```python
from build123d import *

# Parameters (mm, degrees)
F1_DEPTH = 5
F2_R     = 3
F3_DEPTH = 25
F4_SIZE  = 0.6


with BuildPart() as f1:
    # F0 (on Front) → F1 (new body)
    with BuildSketch(Plane.XZ):
        Polygon((2.886751, -5), (5.773503, 0), (2.886751, 5), (-2.886751, 5), (-5.773503, 0), (-2.886751, -5), align=None)
    extrude(amount=F1_DEPTH)

    # F2 (on face) → F3 (join)
    with BuildSketch(Plane.XZ.offset(5)):
        Circle(F2_R)
    extrude(amount=F3_DEPTH)

    # F4
    f4_edges = [f1.edges().sort_by_distance(p)[0] for p in [
        (-3, -30, 0),
    ]]
    chamfer(f4_edges, length=F4_SIZE)

    # F5 (on Right) → F6 (revolve, cut)
    with BuildSketch(Plane.YZ):
        Polygon((2, -1.535898), (-2, -8.464102), (2, -8.464102), align=None)
    revolve(axis=Axis((0, -5, 0), (0, 1, 0)), mode=Mode.SUBTRACT)


solid = f1.part
```
The model under review builds one solid part; all positions refer to its coordinate system, in mm. A direction names the side the tool comes from. Give positions to 0.01 mm unless a question says otherwise; leave off trailing zeros. Order: outer loops, then holes, each group sorted by start corner. A loop starts at its lowest first (then second) coordinate and runs counter-clockwise, first axis right, second up. Notation, with made-up numbers: (18.25, 32.25) - (73.25, 32.25) arc R17 cw to (73.25, 65.25) - close; hole circle Ø3 at (88, 2.25). An arc over 180 degrees is marked (long way). Use CSV: the item, a comma, the result in double quotes. Start each with the question number.
Q1. Clearance check with flat-ended pins moving along their axes: pin 1 Ø1.5 at (y, z) = (-22, -3.5) entering from -X; pin 2 Ø4 at (y, z) = (-26.5, 4) entering from +X; pin 3 Ø1 at (y, z) = (-12.5, 1) entering from +X. State where each tip first meets the part, or that it passes through.
Q2. Tool access review of faces 1 (the flat face through (0, -2, -5)), 2 (the cylindrical face through (-3, -17, 0)): name each direction out of +Z, -Z, +X, -X, +Y, -Y from which nothing blocks a thin tool from reaching the whole face with its end or side.
Q3. We need section B-B, the plane y = -23.5. Write out the cut boundary in (x, z).
Q4. To check wall thickness, follow line 1 along Y through (x, z) = (1, 3.5); line 2 along X through (y, z) = (-3, 1); line 3 along X through (y, z) = (-20.5, 1.75). State the ranges of each line that lie inside material, in increasing order. Write a range as [from, to].
Q5. We need section A-A, the plane y = -4. Write out the cut boundary in (x, z), and give its area (3 significant figures).
Outcome:
1,pin 1,"stops at x = -1.2"
1,pin 2,"stops at x = 2.24"
1,pin 3,"stops at x = 2.96"
2,face 1,"-Z, +X, -X, +Y, -Y"
2,face 2,"-Y"
3,outline,"circle Ø6 at (0, 0)"
4,line 1,"y = [-5, 0]"
4,line 2,"x = [-5.2, 5.2]"
4,line 3,"x = [-2.44, 2.44]"
5,outline,"(-5.77, 0) - (-2.89, -5) - (2.89, -5) - (5.77, 0) - (2.89, 5) - (-2.89, 5) - close"
5,area,"86.6 mm^2"
